For this review, take the finished solid that the model builds, in its own axes (mm). Face numbers are marked on the shaded views. A direction names the side the tool comes from. Give positions to 0.01 mm unless a question says otherwise; leave off trailing zeros. Write each loop counter-clockwise with the first axis right and the second up, starting at its lowest first coordinate (ties: lowest second). Pieces come first, ordered by that corner, then holes. Notation, with made-up numbers: (44, 60.25) -> (86, 60.25) arc R12 ccw to (86, 64.25) -> close; hole circle Ø9 at (-3, 64). An arc over 180 degrees is marked (long way). Return JSON: item names as keys, results as strings.
from build123d import *

# Parameters (mm, degrees)
F1_DEPTH = 10
F3_DEPTH = 2.5


with BuildPart() as f1:
    # F0 (on Top) → F1 (new body)
    with BuildSketch(Plane.XY):
        Polygon((-7.990857, 17.500017), (-8, 20), (-20, 20), (-20, 8), (-17.5, 8), (-17.5, 11.880315), (-14.5, 11.880315), (-14.5, 0), (0, 0), (0, 14.500017), (-12, 14.500017), (-12, 17.500017), align=None)
    extrude(amount=-F1_DEPTH)

    # F2 (on face) → F3 (cut)
    with BuildSketch(Plane.XY):
        with BuildLine():
            Line((0, 0), (0, 10))
            ThreePointArc((0, 10), (-7.071068, 7.071068), (-10, 0))
            Line((-10, 0), (0, 0))
        make_face()
    extrude(amount=-F3_DEPTH, mode=Mode.SUBTRACT)

    # F4: F1 across plane


with BuildPart() as f1_1:
    add(f1.part)
    add(f1.part.mirror(Plane.YZ))

    # F5: F1 across plane


with BuildPart() as f1_2:
    add(f1_1.part)
    add(f1_1.part.mirror(Plane.XZ))


solid = f1_2.part
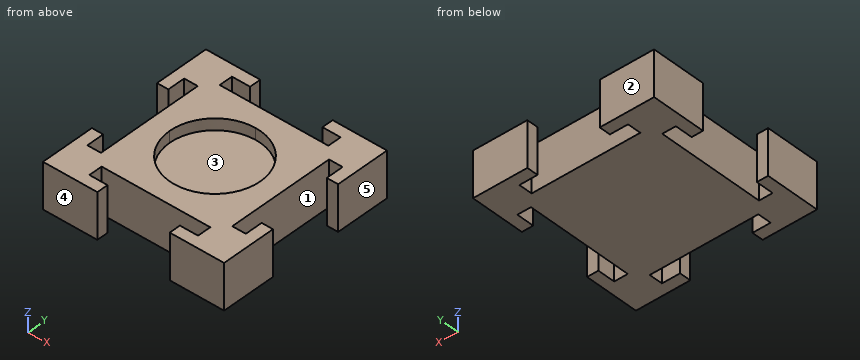
1. To check wall thickness, follow probe 1 along X at (y, z) = (9.5, -6.5); probe 2 along Y at (x, z) = (6, -1.75). State the ranges of each line that lie inside material, in increasing order.
Results found:
{"probe 1": "x = -20 to -17.5, -14.5 to 14.5, 17.5 to 20", "probe 2": "y = -14.5 to -8, 8 to 14.5"}
2. Add section A-A, the plane x = -11.5. State the section outline as (y, z) points, plus the area to 3 significant figures.
Results found:
{"outline": "(-20, -10) -> (-17.5, -10) -> (-17.5, 0) -> (-20, 0) -> close; (-14.5, -10) -> (14.5, -10) -> (14.5, 0) -> (-14.5, 0) -> close; (17.5, -10) -> (20, -10) -> (20, 0) -> (17.5, 0) -> close", "area": "340 mm²"}
3. Add section C-C, the plane y = 2. State the section outline as (x, z) points, plus the area to 3 significant figures.
Results found:
{"outline": "(-14.5, -10) -> (14.5, -10) -> (14.5, 0) -> (9.8, 0) -> (9.8, -2.5) -> (-9.8, -2.5) -> (-9.8, 0) -> (-14.5, 0) -> close", "area": "241 mm²"}
4. Add section B-B, the plane x = 6. State the section outline as (y, z) points, plus the area to 3 significant figures.
Results found:
{"outline": "(-14.5, -10) -> (14.5, -10) -> (14.5, 0) -> (8, 0) -> (8, -2.5) -> (-8, -2.5) -> (-8, 0) -> (-14.5, 0) -> close", "area": "250 mm²"}
5. For the marked faces 1 and 2, list the 3-axis set-ups (+Z, -Z, +X, -X, +Y, -Y) from which the entire face can be reached by the end or side of a thin tool; tool diameter is ignored.
Results found:
{"face 1": "+Z, -Z", "face 2": "+Z, -Z, +X, -X, +Y"}
6. The part is to be moulded in two halves that separate along X. For the marked faces 3, 4 and 5, say which applies: +X half, -X half, draft (parallel to the pull), parting line (faces both ways), or undercut.
Results found:
{"face 3": "undercut", "face 4": "draft", "face 5": "+X half"}
7. For pin 1 (4 mm diameter, centred on x = -0.5, z = -2, fed in from +Y); pin 2 (1 mm diameter, centred on x = -6.5, z = -3.5, fed in from -Y); pin 3 (6 mm diameter, centred on x = -3.5, y = -1.5, fed in from +Z), all flat-tipped, find the tip position at first contact; note any pin that passes through.
Results found:
{"pin 1": "stops at y = 14.5", "pin 2": "stops at y = -14.5", "pin 3": "stops at z = -2.5"}
